Input: part model. Units: mm. Frame: model coordinates. Face numbers are marked on the shaded views. A direction names the side the tool comes from. Round coordinates to 2 decimals unless told otherwise and drop trailing zeros. Order: outer loops, then holes, each group sorted by start corner. A loop starts at its lowest first (then second) coordinate and runs counter-clockwise, first axis right, second up. Notation, with made-up numbers: M 67,-8.5 L 121,-8.5 A8 cw 121,-0.5 Z; hole C 2.5,54 d2. An arc over 180 degrees is marked long. One line per question, with ' | ' between items.
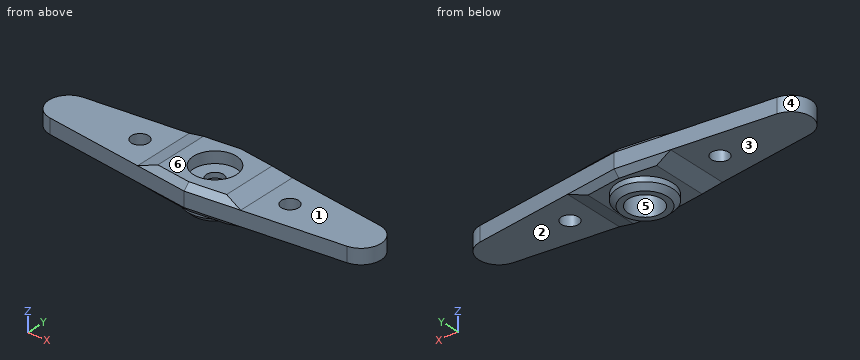
```python
from build123d import *
from OCP.BRepFilletAPI import BRepFilletAPI_MakeChamfer

# Parameters (mm, degrees)
EXTRUDE_1_DEPTH     = 2.6
SKETCH_8_R          = 1.4999999999999987
CUT_EXTRUDE_4_DEPTH = 30.833035380262615
EXTRUDE_2_DEPTH     = 1
CHAMFER_1_SIZE      = 1
CHAMFER_2_SIZE      = 1
CHAMFER_2_SIZE_2    = 3
EXTRUDE_3_DEPTH     = 1
SKETCH_3_R          = 1.5
CUT_EXTRUDE_1_DEPTH = 31.073410182418638
SKETCH_4_R          = 3.75
CUT_EXTRUDE_2_DEPTH = 2
CHAMFER_3_SIZE      = 1
CHAMFER_4_SIZE      = 1
CHAMFER_4_SIZE_2    = 3
SKETCH_6_R          = 4.8
EXTRUDE_4_DEPTH     = 1.8000000000000007
CHAMFER_5_SIZE      = 0.9
SKETCH_7_R          = 2.9
CUT_EXTRUDE_3_DEPTH = 3.5


with BuildPart() as part:
    # ｽｹｯﾁ1 → ﾎﾞｽ - 押し出し1 (new body)
    with BuildSketch(Plane.XY):
        with BuildLine():
            Line((8e-16, 6.5), (25.905749403157248, 3.4764015046938295))
            ThreePointArc((25.905749403157248, 3.4764015046938295), (28.999999999999996, 6.4e-16), (25.905749403157248, -3.476401504693828))
            Line((25.905749403157248, -3.476401504693828), (8e-16, -6.5))
            Line((8e-16, -6.5), (-25.905749403157248, -3.476401504693854))
            ThreePointArc((-25.905749403157248, -3.476401504693854), (-29.000000000000018, -6.03e-15), (-25.905749403157248, 3.4764015046938423))
            Line((-25.905749403157248, 3.4764015046938423), (8e-16, 6.5))
        make_face()
    extrude(amount=EXTRUDE_1_DEPTH)

    # ｽｹｯﾁ8 → ｶｯﾄ - 押し出し4 (cut, through all)
    with BuildSketch(Plane.XY.offset(2.6)):
        with Locations((13.1, 0)):
            Circle(SKETCH_8_R)
        with Locations((-13.1, -1.6e-15)):
            Circle(SKETCH_8_R)
    extrude(amount=-CUT_EXTRUDE_4_DEPTH, mode=Mode.SUBTRACT)

    # ｽｹｯﾁ2 → ﾎﾞｽ - 押し出し2 (add)
    with BuildSketch(Plane.XY.offset(2.6)):
        Polygon((-9.000000000000002, 5.4495618893604005), (-9.000000000000002, -5.449561889360406), (8e-16, -6.5), (9, -5.4495618893604), (9, 5.449561889360396), (8e-16, 6.5), align=None)
    extrude(amount=EXTRUDE_2_DEPTH)

    # 面取り1
    chamfer_1_edges = [part.edges().sort_by_distance(p)[0] for p in [
        (4.500000000000001, -5.9747809446802, 3.6),
        (-4.500000000000001, -5.974780944680203, 3.6),
        (-4.5, 5.9747809446802, 3.6),
        (4.5, 5.974780944680198, 3.6),
    ]]
    chamfer(chamfer_1_edges, length=CHAMFER_1_SIZE)

    # 面取り2
    chamfer_2_edges_1 = [part.edges().sort_by_distance(p)[0] for p in [
        (9, 0, 3.6),
    ]]
    chamfer_2_side_1 = [part.faces().sort_by_distance(p)[0] for p in [
        (9, 0, 3.58),
    ]]
    chamfer_2_edges_2 = [part.edges().sort_by_distance(p)[0] for p in [
        (-9.000000000000002, -8.9e-16, 3.6),
    ]]
    chamfer_2_side_2 = [part.faces().sort_by_distance(p)[0] for p in [
        (-8.980000000000002, -8.9e-16, 3.6),
    ]]
    chamfer_2 = BRepFilletAPI_MakeChamfer(part.part.solid().wrapped)
    for e in chamfer_2_edges_1:
        chamfer_2.Add(CHAMFER_2_SIZE - 0.0001, CHAMFER_2_SIZE_2 - 0.0001, e.wrapped, chamfer_2_side_1[0].wrapped)
    for e in chamfer_2_edges_2:
        chamfer_2.Add(CHAMFER_2_SIZE_2 - 0.0001, CHAMFER_2_SIZE - 0.0001, e.wrapped, chamfer_2_side_2[0].wrapped)
    add(Compound.cast(chamfer_2.Shape()), mode=Mode.REPLACE)  # a hair under: the kernel refuses the full size

    # ｽｹｯﾁ5 → ﾎﾞｽ - 押し出し3 (add)
    with BuildSketch(Plane(origin=(0, 0, 0), x_dir=(-1, 0, 0), z_dir=(0, 0, -1))):
        Polygon((8.999999999999998, 5.449561889360397), (9, -5.449561889360403), (-8e-16, -6.5), (-9, -5.449561889360396), (-9, 5.449561889360396), (-8e-16, 6.5), align=None)
    extrude(amount=EXTRUDE_3_DEPTH)

    # ｽｹｯﾁ3 → ｶｯﾄ - 押し出し1 (cut, through all)
    with BuildSketch(Plane.XY.offset(3.6)):
        Circle(SKETCH_3_R)
    extrude(amount=-CUT_EXTRUDE_1_DEPTH, mode=Mode.SUBTRACT)

    # ｽｹｯﾁ4 → ｶｯﾄ - 押し出し2 (cut)
    with BuildSketch(Plane.XY.offset(3.6)):
        Circle(SKETCH_4_R)
    extrude(amount=-CUT_EXTRUDE_2_DEPTH, mode=Mode.SUBTRACT)

    # 面取り3
    chamfer_3_edges = [part.edges().sort_by_distance(p)[0] for p in [
        (-4.499999999999998, 5.974780944680198, -1),
        (4.5, 5.974780944680198, -1),
        (4.500000000000001, -5.974780944680198, -1),
        (-4.5, -5.974780944680202, -1),
    ]]
    chamfer(chamfer_3_edges, length=CHAMFER_3_SIZE)

    # 面取り4
    chamfer_4_edges_1 = [part.edges().sort_by_distance(p)[0] for p in [
        (9, 0, -1),
    ]]
    chamfer_4_side_1 = [part.faces().sort_by_distance(p)[0] for p in [
        (9, 0, -0.98),
    ]]
    chamfer_4_edges_2 = [part.edges().sort_by_distance(p)[0] for p in [
        (-8.999999999999998, -1.78e-15, -1),
    ]]
    chamfer_4_side_2 = [part.faces().sort_by_distance(p)[0] for p in [
        (-8.979999999999999, -1.78e-15, -1),
    ]]
    chamfer_4 = BRepFilletAPI_MakeChamfer(part.part.solid().wrapped)
    for e in chamfer_4_edges_1:
        chamfer_4.Add(CHAMFER_4_SIZE - 0.0001, CHAMFER_4_SIZE_2 - 0.0001, e.wrapped, chamfer_4_side_1[0].wrapped)
    for e in chamfer_4_edges_2:
        chamfer_4.Add(CHAMFER_4_SIZE_2 - 0.0001, CHAMFER_4_SIZE - 0.0001, e.wrapped, chamfer_4_side_2[0].wrapped)
    add(Compound.cast(chamfer_4.Shape()), mode=Mode.REPLACE)  # a hair under: the kernel refuses the full size

    # ｽｹｯﾁ6 → ﾎﾞｽ - 押し出し4 (add)
    with BuildSketch(Plane(origin=(0, 0, -1), x_dir=(-1, 0, 0), z_dir=(0, 0, -1))):
        Circle(SKETCH_6_R)
    extrude(amount=EXTRUDE_4_DEPTH)

    # 面取り5
    chamfer_5_edges = [part.edges().sort_by_distance(p)[0] for p in [
        (4.800000000000001, -2.88e-15, -2.8000000000000007),
    ]]
    chamfer(chamfer_5_edges, length=CHAMFER_5_SIZE)

    # ｽｹｯﾁ7 → ｶｯﾄ - 押し出し3 (cut)
    with BuildSketch(Plane(origin=(0, 0, -2.8000000000000007), x_dir=(-1, 0, 0), z_dir=(0, 0, -1))):
        Circle(SKETCH_7_R)
    extrude(amount=-CUT_EXTRUDE_3_DEPTH, mode=Mode.SUBTRACT)


solid = part.part
```
Item 1: Mould query, pull axis Y, two halves, no side actions, for the marked faces 4, 5 and 6. Classes: +Y half, -Y half, draft (parallel to the pull), parting line (faces both ways), or undercut.
Report:
face 4: parting line | face 5: undercut | face 6: draft
Item 2: Access query for the marked faces 1, 2 and 3. Directions: +Z, -Z, +X, -X, +Y, -Y. A direction counts if a zero-diameter tool reaches every point of the face in a straight line with its end or side. Return the directions, or none.
Report:
face 1: +Z, +X, +Y, -Y | face 2: -Z, +X, +Y, -Y | face 3: -Z, -X, +Y, -Y
Item 3: Section query A-A, the plane x = -13.1. Return loops of the section in (y, z), plus the area to 3 significant figures.
Report:
outline: M -4.97,0 L -1.5,0 L -1.5,2.6 L -4.97,2.6 Z; M 1.5,0 L 4.97,0 L 4.97,2.6 L 1.5,2.6 Z | area: 18.0 mm²
Item 4: Section query B-B, the plane y = 0. Give the number of separate pieces and of enclosed holes in the cut face, plus the area to 3 significant figures.
Report:
separate pieces: 4 | enclosed holes: 0 | area: 144 mm²
Item 5: Section query C-C, the plane x = 5.5. Return loops of the section in (y, z), plus the area to 3 significant figures.
Report:
outline: M -5.86,0 L -4.85,-1 L 4.85,-1 L 5.86,0 L 5.86,2.6 L 4.85,3.6 L -4.85,3.6 L -5.86,2.6 Z | area: 51.9 mm²
Item 6: First-contact query: pin 1 (7 mm diameter, centred on x = 0, y = 0, fed in from +Z); pin 2 (5.5 mm diameter, centred on x = 14.5, y = 2.5, fed in from -Z); pin 3 (1 mm diameter, centred on y = -1, z = -2, fed in from -X). Flat tips, straight axial feed; report the tip coordinate or a pass-through.
Report:
pin 1: z = 1.6 | pin 2: z = 0 | pin 3: x = -4.77
Item 7: Line query: line 1 along Z through (x, y) = (-21.5, 2.5); line 2 along Y through (x, z) = (-9, 2); line 3 along Y through (x, z) = (-13.1, 2). Output: solid intervals per line, ascending. Write a range as from..to.
Report:
line 1: 0..2.6 | line 2: -5.45..5.45 | line 3: -4.97..-1.5, 1.5..4.97
